Input: part model. Units: mm. Frame: model coordinates. A direction names the side the tool comes from. Give positions to 0.01 mm unless a question says otherwise; leave off trailing zeros. Write each loop counter-clockwise with the first axis right and the second up, starting at its lowest first coordinate (ties: lowest second). Pieces come first, ordered by that corner, then holes. Notation, with made-up numbers: (-15, 20) - (-10, 20) arc R20 ccw to (-10, 31) - close; hole circle Ø1 at (-10.75, -0.75). An arc over 180 degrees is marked (long way). Answer as a JSON object with one key per item and string values. Group by question number.
Autodesk Inventor part; units mm, degrees
ref_plane "Arbeitsebene1" through (0, 0, 0) normal (1, 0, 0) x (0, 1, 0)
ref_plane "XZ Plane" through (0, 0, 0) normal (0, 1, 0) x (-1, 0, 0)
ref_plane "XY Plane" through (0, 0, 0) normal (0, 0, 1) x (1, 0, 0)
sketch "Skizze1" plane through (0, 0, 0) normal (0, 0, 1) x (-1, 0, 0)
  circle A0 centre (0, 0) radius 22.5
  dimension "d0" = 45
extrude "Extrusion1" add sketch "Skizze1" against normal blind 20
sketch "Skizze3" plane through (0, 0, 0) normal (0, 0, 1) x (1, 0, 0)
  circle A0 centre (0, 0) radius 15
  dimension "d3" = 30
extrude "Extrusion2" add sketch "Skizze3" along normal blind 20
ref_plane "Arbeitsebene1" through (0, 0, 0) normal (1, 0, 0) x (0, 1, 0)
sketch "Skizze5" plane through (0, 0, 0) normal (1, 0, 0) x (0, 1, 0)
  line L0 (-22.5, -20) -> (22.5, -20)
  line L1 (0, -20) -> (0, 20)
  line L2 (15, 20) -> (-15, 20)
  line L3 (10, 20) -> (10, 1.8057) construction
  line L4 (10, 2.5) -> (10, 12.5)
  line L5 (15, 2.5) -> (15, 12.5)
  line L6 (15, 0) -> (15, 20)
  arc A0 (15, 12.5) -> (15, 2.5) centre (15, 7.5) ccw
  point P0 (0, 0)
  point P1 (10, 7.5)
  dimension "d8" = 20
  dimension "d10" = 7.5
  dimension "d13" = 5
revolve "Umdrehung1" cut sketch "Skizze5" angle 360 about axis through (0, 0, -20) along (0, 0, 1)
properties part number "7"
1) Line query: line 1 along Z through (x, y) = (-12.5, -8); line 2 along Z through (x, y) = (15, -6); line 3 along Z through (x, y) = (11.5, -4). Output: solid intervals per line, ascending. Write a range as from..to.
2) Reachability of faces 1 (the face through (0, 0, 20)), 2 (the face through (-14.985, -0.66, 16.197)) from +Z, -Z, +X, -X, +Y, -Y: full face, straight path, thin tool, end or side. Return the list, or none.
3) Cut plane A-A on y = 0. Return the cut outline in (x, z).
4) Cut plane C-C on y = 19. Return the cut outline in (x, z), and give its area (3 significant figures).
5) Pin query (flat end, axial travel): P1, Ø8, axis at x = -17, z = -3.5, coming from the -Y side; P2, Ø3, axis at y = -7.5, z = -1, coming from the +X side; P3, Ø10, axis at x = -5.5, z = -13.5, coming from the +Y side; P4, Ø5, axis at y = 1.5, z = -9.5, coming from the -X side. Return the tip coordinate at first contact, or that it passes through.
Filled in:
{
 "1": {"line 1": "z = -20..2.5, 12.5..20", "line 2": "z = -20..0", "line 3": "z = -20..3.37, 11.63..20"},
 "2": {"face 1": "+Z, +X, -X, +Y, -Y", "face 2": "+Z"},
 "3": {"outline": "(-22.5, -20) - (22.5, -20) - (22.5, 0) - (15, 0) - (15, 2.5) arc R5 cw to (15, 12.5) - (15, 20) - (-15, 20) - (-15, 12.5) arc R5 cw to (-15, 2.5) - (-15, 0) - (-22.5, 0) - close"},
 "4": {"outline": "(-12.05, -20) - (12.05, -20) - (12.05, 0) - (-12.05, 0) - close", "area": "482 mm²"},
 "5": {"P1": "stops at y = -18.36", "P2": "stops at x = 21.69", "P3": "stops at y = 22.49", "P4": "stops at x = -22.5"}
}
